Build history of the part. All positions in model axes, mm. A direction names the side the tool comes from. Coordinates: 2 decimals unless noted, no trailing zeros. Loops run counter-clockwise (first coordinate to the right, second up) from the corner with the lowest first, then second, coordinate; pieces in that order, holes last.
Item 1: Mould opens along Y. For faces 1 (the face through (46.48, -5.76, 7.01)), 2 (the face through (-45, 0, 8)), 3 (the face through (33, 8.1, 18)) say: released by +Y, released by -Y, zero draft, split by the parting line, or undercut.
Item 2: Cut at D-D (x = 17). List the corners of the cut face in (y, z), and give its area (3 significant figures).
Item 3: Cut at B-B (y = 5). Count the separate pieces of the cut face and the enclosed holes in it, and give its area (3 significant figures).
Item 4: 3-axis set-ups, long thin cutter, end or side, ignore diameter. For faces 4 (the face through (12, 0.95, 15)), 5 (the face through (46, 0, 13)), 6 (the face through (45, 0, 8)), 7 (the face through (-46.52, 4.24, 7.01)): which of +Z, -Z, +X, -X, +Y, -Y reach the whole face in a straight line?
Item 5: Cut at A-A (x = 0.32). List the corners of the cut face in (y, z), and give its area (3 significant figures).
Item 6: Drill centre lines: line 1 along X through (y, z) = (8.75, 6.5); line 2 along Y through (x, z) = (-46.1, 8); line 3 along X through (y, z) = (-1, 7) (3 decimals). Where is each one in solid material? Low to high.
Item 7: Flat gauge pins, fed straight in: pin 1 (4 mm diameter, centred on y = 5, z = 18.5, fed in from +X); pin 2 (1.5 mm diameter, centred on x = -32, y = 2, fed in from +Z); pin 3 (10 mm diameter, centred on x = 24.5, z = 24, fed in from -Y). Where does each tip first touch, or does it go through?
from build123d import *
from OCP.BRepFilletAPI import BRepFilletAPI_MakeChamfer

# Parameters (mm, degrees)
SCHIZZO1_W                   = 96
SCHIZZO1_H                   = 20
SCHIZZO1_R                   = 1
SCHIZZO1_R_2                 = 1.25
ESTRUSIONE_ESTRUSIONE1_DEPTH = 3
SCHIZZO2_W                   = 3
SCHIZZO2_H                   = 20
ESTRUSIONE_ESTRUSIONE2_DEPTH = 10
SCHIZZO3_R                   = 1.25
TAGLIO_ESTRUSIONE1_DEPTH     = 98.390964673
SCHIZZO4_W                   = 12
SCHIZZO4_H                   = 4
ESTRUSIONE_ESTRUSIONE3_DEPTH = 27
RACCORDO1_R                  = 6
SCHIZZO5_R                   = 4.2
TAGLIO_ESTRUSIONE2_DEPTH     = 60.427350606
SMUSSO1_SIZE                 = 10.775435457
SMUSSO1_SIZE_2               = 1.9
SCHIZZO6_W                   = 5
SCHIZZO6_H                   = 3
ESTRUSIONE_ESTRUSIONE4_DEPTH = 23.5
RACCORDO2_R                  = 2.5
SCHIZZO7_R                   = 1.5
TAGLIO_ESTRUSIONE3_DEPTH     = 59.297534253
SMUSSO2_SIZE                 = 5
SMUSSO2_SIZE2                = 8.660254038


with BuildPart() as part:
    # Schizzo1 → Estrusione-Estrusione1 (new body)
    with BuildSketch(Plane.XY):
        Rectangle(SCHIZZO1_W, SCHIZZO1_H)
        with Locations((20.125, 0)):
            Circle(SCHIZZO1_R, mode=Mode.SUBTRACT)
        with Locations((-40.32, 7.62)):
            Circle(SCHIZZO1_R_2, mode=Mode.SUBTRACT)
        with Locations((0.32, 7.62)):
            Circle(SCHIZZO1_R_2, mode=Mode.SUBTRACT)
        with Locations((0.32, -7.62)):
            Circle(SCHIZZO1_R_2, mode=Mode.SUBTRACT)
        with Locations((-40.32, -7.62)):
            Circle(SCHIZZO1_R_2, mode=Mode.SUBTRACT)
    extrude(amount=ESTRUSIONE_ESTRUSIONE1_DEPTH)

    # Schizzo2 → Estrusione-Estrusione2 (add)
    with BuildSketch(Plane.XY.offset(3)):
        with Locations((-46.5, 0)):
            Rectangle(SCHIZZO2_W, SCHIZZO2_H)
        with Locations((46.5, 0)):
            Rectangle(SCHIZZO2_W, SCHIZZO2_H)
    extrude(amount=ESTRUSIONE_ESTRUSIONE2_DEPTH)

    # Schizzo3 → Taglio-Estrusione1 (cut, through all)
    with BuildSketch(Plane.ZY.offset(48)):
        with Locations((8, -5)):
            Circle(SCHIZZO3_R)
        with Locations((8, 5)):
            Circle(SCHIZZO3_R)
    extrude(amount=-TAGLIO_ESTRUSIONE1_DEPTH, mode=Mode.SUBTRACT)

    # Schizzo4 → Estrusione-Estrusione3 (add)
    with BuildSketch(Plane.XY.offset(3)):
        with Locations((33, -6.1)):
            Rectangle(SCHIZZO4_W, SCHIZZO4_H)
        with Locations((33, 6.1)):
            Rectangle(SCHIZZO4_W, SCHIZZO4_H)
    extrude(amount=ESTRUSIONE_ESTRUSIONE3_DEPTH)

    # Raccordo1
    raccordo1_edges = [part.edges().sort_by_distance(p)[0] for p in [
        (27, 6.1, 30),
        (39, 6.1, 30),
        (39, -6.1, 30),
        (27, -6.1, 30),
    ]]
    fillet(raccordo1_edges, radius=RACCORDO1_R - 0.0001)  # a hair under: the kernel refuses the full size

    # Schizzo5 → Taglio-Estrusione2 (cut, through all)
    with BuildSketch(Plane(origin=(0, 8.1, 0), x_dir=(1, 0, 0), z_dir=(0, 1, 0))):
        with Locations(Location((33, -24, 0), (0, 0, 180))):
            Circle(SCHIZZO5_R)
    extrude(amount=-TAGLIO_ESTRUSIONE2_DEPTH, mode=Mode.SUBTRACT)

    # Smusso1
    smusso1_edges_1 = [part.edges().sort_by_distance(p)[0] for p in [
        (33, -8.1, 3),
    ]]
    smusso1_side_1 = [part.faces().sort_by_distance(p)[0] for p in [
        (33, -8.1, 3.038),
    ]]
    smusso1_edges_2 = [part.edges().sort_by_distance(p)[0] for p in [
        (33, 8.1, 3),
    ]]
    smusso1_side_2 = [part.faces().sort_by_distance(p)[0] for p in [
        (33, 8.138, 3),
    ]]
    smusso1 = BRepFilletAPI_MakeChamfer(part.part.solid().wrapped)
    for e in smusso1_edges_1:
        smusso1.Add(SMUSSO1_SIZE - 0.0001, SMUSSO1_SIZE_2 - 0.0001, e.wrapped, smusso1_side_1[0].wrapped)
    for e in smusso1_edges_2:
        smusso1.Add(SMUSSO1_SIZE_2 - 0.0001, SMUSSO1_SIZE - 0.0001, e.wrapped, smusso1_side_2[0].wrapped)
    add(Compound.cast(smusso1.Shape()), mode=Mode.REPLACE)  # a hair under: the kernel refuses the full size

    # Schizzo6 → Estrusione-Estrusione4 (add)
    with BuildSketch(Plane.XY.offset(3)):
        with Locations((12.525, 2.45)):
            Rectangle(SCHIZZO6_W, SCHIZZO6_H)
        with Locations((12.525, -2.45)):
            Rectangle(SCHIZZO6_W, SCHIZZO6_H)
    extrude(amount=ESTRUSIONE_ESTRUSIONE4_DEPTH)

    # Raccordo2
    raccordo2_edges = [part.edges().sort_by_distance(p)[0] for p in [
        (15.025, -2.45, 26.5),
        (10.025, -2.45, 26.5),
        (15.025, 2.45, 26.5),
        (10.025, 2.45, 26.5),
    ]]
    fillet(raccordo2_edges, radius=RACCORDO2_R - 0.0001)  # a hair under: the kernel refuses the full size

    # Schizzo7 → Taglio-Estrusione3 (cut, through all)
    with BuildSketch(Plane(origin=(0, 3.95, 0), x_dir=(1, 0, 0), z_dir=(0, 1, 0))):
        with Locations(Location((12.525, -24, 0), (0, 0, 180))):
            Circle(SCHIZZO7_R)
    extrude(amount=-TAGLIO_ESTRUSIONE3_DEPTH, mode=Mode.SUBTRACT)

    # Smusso2
    smusso2_edges = [part.edges().sort_by_distance(p)[0] for p in [
        (12.525, 3.95, 3),
        (12.525, -3.95, 3),
    ]]
    smusso2_side = [part.faces().sort_by_distance(p)[0] for p in [
        (-2.939038544, 0, 3),
    ]]
    chamfer(smusso2_edges, length=SMUSSO2_SIZE, length2=SMUSSO2_SIZE2, reference=smusso2_side[0])


solid = part.part
Filled sheet:
1. face 1: undercut
1. face 2: zero draft
1. face 3: released by +Y
2. outline: (-10, 0) - (10, 0) - (10, 3) - (-10, 3) - close
2. area: 60.0 mm2
3. separate pieces: 3
3. enclosed holes: 1
3. area: 620 mm2
4. face 4: +Z
4. face 5: +Z, +X, +Y, -Y
4. face 6: +Z, +Y, -Y
4. face 7: -X
5. outline: (-10, 0) - (-8.87, 0) - (-8.87, 3) - (-10, 3) - close; (-6.37, 0) - (6.37, 0) - (6.37, 3) - (-6.37, 3) - close; (8.87, 0) - (10, 0) - (10, 3) - (8.87, 3) - close
5. area: 45.0 mm2
6. line 1: x = -48 to -45, 27 to 39, 45 to 48
6. line 2: y = -10 to -6.25, -3.75 to 3.75, 6.25 to 10
6. line 3: x = -48 to -45, 10.025 to 15.025, 45 to 48
7. pin 1: stops at x = 39
7. pin 2: stops at z = 3
7. pin 3: stops at y = -8.1
